from build123d import *

# Parameters (mm, degrees)
SKETCH1_W                   = 50.8
SKETCH1_H                   = 25.4
BOSS_EXTRUDE1_DEPTH         = 20
BOSS_EXTRUDE2_DEPTH         = 25.4
FILLET1_R                   = 10
FILLET2_R                   = 2
SKETCH3_R                   = 5
CUT_EXTRUDE1_DEPTH          = 40.184818489
TAP_DRILL_FOR_M2X0_4_TAP1_D = 1.6


with BuildPart() as part:
    # Sketch1 → Boss-Extrude1 (new body)
    with BuildSketch(Plane(origin=(0, 0, 0), x_dir=(1, 0, 0), z_dir=(0, 1, 0))):
        Rectangle(SKETCH1_W, SKETCH1_H)
    extrude(amount=BOSS_EXTRUDE1_DEPTH)

    # Sketch2 → Boss-Extrude2 (add, through all)
    with BuildSketch(Plane.XY.offset(12.7)):
        with BuildLine():
            Line((3.464101615, 22), (25.4, 22))
            Line((25.4, 22), (25.4, 27))
            Line((25.4, 27), (9.539392014, 27))
            ThreePointArc((9.539392014, 27), (3.478061726, 33.375664597), (-5.274899627, 32.495612628))
            Line((-5.274899627, 32.495612628), (-25.4, 20))
            Line((-25.4, 20), (-4.8e-08, 20))
            ThreePointArc((-4.8e-08, 20), (-2.828427108, 26.828427142), (4, 24))
            ThreePointArc((4, 24), (3.863703305, 22.96472382), (3.464101615, 22))
        make_face()
    extrude(amount=-BOSS_EXTRUDE2_DEPTH)

    # Fillet1
    fillet1_edges = [part.edges().sort_by_distance(p)[0] for p in [
        (9.539392014, 27, 0),
    ]]
    fillet(fillet1_edges, radius=FILLET1_R)

    # Fillet2
    fillet2_edges = [part.edges().sort_by_distance(p)[0] for p in [
        (3.464101615, 22, 0),
    ]]
    fillet(fillet2_edges, radius=FILLET2_R - 0.0001)  # a hair under: the kernel refuses the full size

    # Sketch3 → Cut-Extrude1 (cut, through all)
    with BuildSketch(Plane(origin=(0, 27, 0), x_dir=(1, 0, 0), z_dir=(0, 1, 0))):
        with Locations((15.4, 0)):
            Circle(SKETCH3_R)
    extrude(amount=CUT_EXTRUDE1_DEPTH, mode=Mode.SUBTRACT)

    # Tap Drill for M2x0.4 Tap1 (through all)
    with Locations(Plane(origin=(0, 27, 0), x_dir=(1, 0, 0), z_dir=(0, 1, 0))):
        with Locations((15.4, 0)):
            Hole(TAP_DRILL_FOR_M2X0_4_TAP1_D / 2)


solid = part.part
Part model, mm, in its own coordinate system. A direction names the side the tool comes from. Round coordinates to 2 decimals unless told otherwise and drop trailing zeros. Order: outer loops, then holes, each group sorted by start corner. A loop starts at its lowest first (then second) coordinate and runs counter-clockwise, first axis right, second up. Notation, with made-up numbers: (-5.5, 37) -> (27.5, 37) arc R17 ccw to (27.5, 41) -> close; hole circle Ø1 at (34.25, 43). An arc over 180 degrees is marked (long way). Put each result on its own line as item: value.
Q1. Pin check, flat tips, straight feed: pin 1 Ø1.8 at (x, z) = (15.4, 0) entering from +Y; pin 2 Ø12 at (x, z) = (16, -5.5) entering from +Y; pin 3 Ø1 at (x, z) = (-11.5, -4.5) entering from +Y; pin 4 Ø1.3 at (x, z) = (15.4, 0) entering from -Y. Stop position of each tip, or through.
From the geometry:
pin 1: stops at y = 27
pin 2: stops at y = 28.46
pin 3: stops at y = 28.94
pin 4: passes through
Q2. Band-saw the part on B-B (x = 22). Give the cut face in (y, z).
From the geometry:
outline: (0, -12.7) -> (20, -12.7) -> (20, 12.7) -> (0, 12.7) -> close; (22, -12.7) -> (27, -12.7) -> (27, 12.7) -> (22, 12.7) -> close
Q3. Band-saw the part on A-A (z = 0). Give the cut face in (x, y).
From the geometry:
outline: (-25.4, 0) -> (14.6, 0) -> (14.6, 20) -> (0, 20) arc R4 cw (long way) to (4, 24) arc R2 ccw to (6, 22) -> (14.6, 22) -> (14.6, 27) -> (10.4, 27) -> (10.4, 28.23) arc R10 cw to (7.6, 30.5) arc R10 ccw to (-5.27, 32.5) -> (-25.4, 20) -> close; (16.2, 0) -> (25.4, 0) -> (25.4, 20) -> (16.2, 20) -> close; (16.2, 22) -> (25.4, 22) -> (25.4, 27) -> (16.2, 27) -> close
Q4. Band-saw the part on C-C (z = 10.5). Give the cut face in (x, y).
From the geometry:
outline: (-25.4, 0) -> (25.4, 0) -> (25.4, 20) -> (0, 20) arc R4 cw (long way) to (4, 24) arc R2 ccw to (6, 22) -> (25.4, 22) -> (25.4, 27) -> (15.2, 27) arc R10 cw to (7.6, 30.5) arc R10 ccw to (-5.27, 32.5) -> (-25.4, 20) -> close
Q5. Wall check: line 1 (Y direction, x = 0, z = 6); line 2 (Z direction, x = 15.4, y = 23.9); line 3 (Y direction, x = 22.5, z = -8.5). Give the ranges that are in metal, low to high. Write a range as [from, to].
From the geometry:
line 1: y = [0, 20], [28, 34]
line 2: z = [-12.7, -0.8], [0.8, 12.7]
line 3: y = [0, 20], [22, 27]
Q6. Band-saw the part on D-D (x = -15). Give the cut face in (y, z).
From the geometry:
outline: (0, -12.7) -> (26.46, -12.7) -> (26.46, 12.7) -> (0, 12.7) -> close
Q7. Pull direction X, two halves, no side cores. Call faces 1 (the face through (25.4, 24, 0)), 2 (the face through (13, 20, 0)), 3 (the face through (4.6, 22.57, -0.18)): pulls with the +X half, pulls with the -X half, needs draft (parallel to the pull), parting line crosses it, or undercut.
From the geometry:
face 1: pulls with the +X half
face 2: needs draft
face 3: undercut
Q8. Tool access for faces 4 (the face through (10.4, 27.5, -0.1)), 5 (the face through (13, 22, 0)), 6 (the face through (-15.197, 26.335, 0.178)): list every direction of +Z, -Z, +X, -X, +Y, -Y with a clear straight run to the whole face (end or side of a thin tool).
From the geometry:
face 4: +X, +Y
face 5: +Z, -Z, +X
face 6: +Z, -Z, -X, +Y
